Verification items for the finished model (mm, model axes). Coordinates: 2 decimals unless noted, no trailing zeros. Order: outer loops, then holes, each group sorted by start corner. A loop starts at its lowest first (then second) coordinate and runs counter-clockwise, first axis right, second up. Notation, with made-up numbers: (38, 35.5) -> (79, 35.5) arc R21 cw to (79, 59.5) -> close; hole circle Ø7 at (67, 27). An arc over 180 degrees is marked (long way). Answer as CSV lines item,"result".
Autodesk Inventor part; units mm, degrees
ref_plane "РабПлоскость1" through (30, 0, 0) normal (1, 0, 0) x (0, 1, 0)
ref_plane "YZ Plane" through (0, 0, 0) normal (1, 0, 0) x (0, 1, 0)
ref_plane "XZ Plane" through (0, 0, 0) normal (0, 1, 0) x (-1, 0, 0)
sketch "Эскиз1" plane through (0, 0, 0) normal (0, 0, 1) x (1, 0, 0)
  circle A0 centre (0, 0) radius 20
  circle A1 centre (0, 0) radius 30
  dimension "d0" = 40
  dimension "d1" = 10
extrude "Выдавливание1" add sketch "Эскиз1" along normal mid plane 90
ref_plane "РабПлоскость1" through (30, 0, 0) normal (1, 0, 0) x (0, 1, 0)
sketch "Эскиз4" plane through (30, 0, 0) normal (1, 0, 0) x (0, 1, 0)
  circle A0 centre (0, 0) radius 5
  dimension "d5" = 10
extrude "Выдавливание2" add sketch "Эскиз4" against normal up to surface
sketch "Эскиз6" plane through (30, 0, 0) normal (1, 0, 0) x (0, 0, -1)
  arc A0 (5, 0) -> (-5, 0) centre (0, 0) ccw
  circle A1 centre (0, 0) radius 4.9989
  point P0 (-10, 0)
  point P1 (10, 0)
extrude "Выдавливание3" add sketch "Эскиз6" along normal blind 10
properties part number "стакан_v1"
Item 1: Section check C-C, the plane z = 0. Record the boundary of the cut face in (x, y).
Answer list:
outline,"(29.58, -5) -> (40, -5) -> (40, 5) -> (29.58, 5) arc R30 ccw (long way) to start; hole circle Ø40 at (0, 0)"
Item 2: Section check A-A, the plane x = 0. Record the boundary of the cut face in (y, z).
Answer list:
outline,"(-30, -45) -> (-20, -45) -> (-20, 45) -> (-30, 45) -> close; (20, -45) -> (30, -45) -> (30, 45) -> (20, 45) -> close"
Item 3: Section check D-D, the plane z = 27.5. Record the boundary of the cut face in (x, y), plus the area to 3 significant figures.
Answer list:
outline,"circle Ø60 at (0, 0); hole circle Ø40 at (0, 0)"
area,"1,570 mm2"
Item 4: Depth check by flat-ended pin: pin 1 Ø8 at (y, z) = (5, -30.5) entering from +X; pin 2 Ø1 at (y, z) = (-8.5, -15.5) entering from -X; pin 3 Ø3 at (y, z) = (-5, 35) entering from -X. Enter the tip coordinate at first touch or a pass-through.
Answer list:
pin 1,"x = 29.98"
pin 2,"x = -28.91"
pin 3,"x = -29.8"
Item 5: Release check for a two-part mould opening along Y. For faces 1 (the cylindrical face through (35, -5, 0)), 2 (the cylindrical face through (35, 5, 0)), 3 (the cylindrical face through (-4.336, 19.524, -0.63)), 4 (the flat face through (6, -20, -45)) record: +Y half, -Y half, draft (parallel to the pull), parting line (faces both ways), or undercut.
Answer list:
face 1,"-Y half"
face 2,"+Y half"
face 3,"undercut"
face 4,"draft"
Item 6: Thickness scan on line 1 (Y direction, x = 0, z = -17); line 2 (Y direction, x = 10.5, z = -11); line 3 (X direction, y = 5, z = 20). Record the ranges inside material, lowest first.
Answer list:
line 1,"-30 to -20, 20 to 30"
line 2,"-28.1 to -17.02, 17.02 to 28.1"
line 3,"-29.58 to -19.36, 19.36 to 29.58"
Item 7: Section check B-B, the plane y = 17. Record the boundary of the cut face in (x, z).
Answer list:
outline,"(-24.72, -45) -> (-10.54, -45) -> (-10.54, 45) -> (-24.72, 45) -> close; (10.54, -45) -> (24.72, -45) -> (24.72, 45) -> (10.54, 45) -> close"
